```python
from build123d import *

# Parameters (mm, degrees)
SKETCH1_W            = 126
SKETCH1_H            = 76
BOSS_EXTRUDE1_DEPTH  = 13
SKETCH2_W            = 126
SKETCH2_H            = 90
BOSS_EXTRUDE2_DEPTH  = 13
FILLET1_R            = 25
SKETCH3_W            = 10
SKETCH3_H            = 25.459891015
BOSS_EXTRUDE3_DEPTH  = 10
SKETCH4_W            = 10
SKETCH4_H            = 13
CUT_EXTRUDE1_DEPTH   = 10
SKETCH8_R            = 25
BOSS_EXTRUDE4_DEPTH  = 38
SKETCH10_R           = 16
CUT_EXTRUDE3_DEPTH   = 38
BOSS_EXTRUDE8_DEPTH  = 25
SKETCH12_W           = 10
SKETCH12_H           = 10
CUT_EXTRUDE4_DEPTH   = 45
SKETCH13_R           = 8.829907476
CUT_EXTRUDE5_DEPTH   = 14
SKETCH14_R           = 7
CUT_EXTRUDE6_DEPTH   = 34
BOSS_EXTRUDE11_DEPTH = 37
CUT_EXTRUDE7_DEPTH   = 37


with BuildPart() as part:
    # Sketch1 → Boss-Extrude1 (new body)
    with BuildSketch(Plane(origin=(0, 0, 0), x_dir=(1, 0, 0), z_dir=(0, 1, 0))):
        with Locations((9.064748201, -38.597122302)):
            Rectangle(SKETCH1_W, SKETCH1_H)
    extrude(amount=BOSS_EXTRUDE1_DEPTH)

    # Sketch2 → Boss-Extrude2 (add)
    with BuildSketch(Plane(origin=(0, 0, 0.597122302), x_dir=(-1, 0, 0), z_dir=(0, 0, -1))):
        with Locations((-9.064748201, 58)):
            Rectangle(SKETCH2_W, SKETCH2_H)
    extrude(amount=-BOSS_EXTRUDE2_DEPTH)

    # Fillet1
    fillet1_edges = [part.edges().sort_by_distance(p)[0] for p in [
        (72.064748201, 103, 7.097122302),
        (-53.935251799, 103, 7.097122302),
    ]]
    fillet(fillet1_edges, radius=FILLET1_R)

    # Sketch3 → Boss-Extrude3 (add)
    with BuildSketch(Plane(origin=(0, 103, 0), x_dir=(1, 0, 0), z_dir=(0, 1, 0))):
        with Locations((9.064748201, -26.32706781)):
            Rectangle(SKETCH3_W, SKETCH3_H)
    extrude(amount=-BOSS_EXTRUDE3_DEPTH)

    # Sketch4 → Cut-Extrude1 (cut)
    with BuildSketch(Plane(origin=(0, 103, 0), x_dir=(1, 0, 0), z_dir=(0, 1, 0))):
        with Locations((9.064748201, -7.097122302)):
            Rectangle(SKETCH4_W, SKETCH4_H)
    extrude(amount=-CUT_EXTRUDE1_DEPTH, mode=Mode.SUBTRACT)

    # Sketch8 → Boss-Extrude4 (add)
    with BuildSketch(Plane.XY.offset(13.597122302)):
        with Locations((9.064748201, 45.775653821)):
            Circle(SKETCH8_R)
    extrude(amount=BOSS_EXTRUDE4_DEPTH)

    # Sketch10 → Cut-Extrude3 (cut)
    with BuildSketch(Plane.XY.offset(51.597122302)):
        with Locations((9.064748201, 45.775653821)):
            Circle(SKETCH10_R)
    extrude(amount=-CUT_EXTRUDE3_DEPTH, mode=Mode.SUBTRACT)

    # Sketch11 → Boss-Extrude8 (add)
    with BuildSketch(Plane.XY.offset(13.597122302)):
        with BuildLine():
            Line((4.064748201, 103), (-5.935251799, 103))
            Line((-5.935251799, 103), (-5.935251799, 65.775653821))
            ThreePointArc((-5.935251799, 65.775653821), (9.064748201, 70.775653821), (24.064748201, 65.775653821))
            Line((24.064748201, 65.775653821), (24.064748201, 103))
            Line((24.064748201, 103), (14.064748201, 103))
            Line((14.064748201, 103), (14.064748201, 93))
            Line((14.064748201, 93), (4.064748201, 93))
            Line((4.064748201, 93), (4.064748201, 103))
        make_face()
    extrude(amount=BOSS_EXTRUDE8_DEPTH)

    # Sketch12 → Cut-Extrude4 (cut)
    with BuildSketch(Plane.XY.offset(39.057013317)):
        with Locations((9.064748201, 98)):
            Rectangle(SKETCH12_W, SKETCH12_H)
    extrude(amount=-CUT_EXTRUDE4_DEPTH, mode=Mode.SUBTRACT)

    # Sketch13 → Cut-Extrude5 (cut)
    with BuildSketch(Plane(origin=(0, 13, 0), x_dir=(1, 0, 0), z_dir=(0, 1, 0))):
        with Locations((-34.808854568, -51.290114298)):
            Circle(SKETCH13_R)
    extrude(amount=-CUT_EXTRUDE5_DEPTH, mode=Mode.SUBTRACT)

    # Sketch14 → Cut-Extrude6 (cut)
    with BuildSketch(Plane(origin=(0, 13, 0), x_dir=(1, 0, 0), z_dir=(0, 1, 0))):
        with Locations((53.064748201, -51.597122302)):
            Circle(SKETCH14_R)
    extrude(amount=-CUT_EXTRUDE6_DEPTH, mode=Mode.SUBTRACT)

    # Sketch17 → Boss-Extrude11 (add, symmetric)
    with BuildSketch(Plane.XY.offset(51.597122302)):
        Polygon((3.660374399, 21.366787731), (13.431056495, 21.159899681), (13.431056495, 13), (3.660374399, 13), align=None)
    extrude(amount=BOSS_EXTRUDE11_DEPTH, both=True)

    # Sketch18 → Cut-Extrude7 (cut, symmetric)
    with BuildSketch(Plane(origin=(13.431056495, 0, 0), x_dir=(0, 0, -1), z_dir=(1, 0, 0))):
        Polygon((-51.597122302, 21.159899681), (-76.597122302, 13), (-88.597122302, 13), (-88.597122302, 23.683887041), align=None)
    extrude(amount=CUT_EXTRUDE7_DEPTH, both=True, mode=Mode.SUBTRACT)


solid = part.part
```
Geometry check sheet. Reference: the model listing, model coordinates, mm. A direction names the side the tool comes from. Coordinates: 2 decimals unless noted, no trailing zeros. Loops run counter-clockwise (first coordinate to the right, second up) from the corner with the lowest first, then second, coordinate; pieces in that order, holes last.
Item 1: Go/stop test with flat-tipped pins: pin 1 Ø15 at (x, y) = (20.5, 57.5) entering from +Z; pin 2 Ø3 at (x, z) = (11, 18) entering from +Y; pin 3 Ø7.5 at (y, z) = (78.5, 21) entering from -X; pin 4 Ø4 at (y, z) = (58.5, 54) entering from -X. Record where each tip stops, or that it passes through.
Item 2: Sectioned sample at A-A, the plane z = 28. Record the boundary of the cut face in (x, y), then the cut area to 3 significant figures.
Item 3: Sectioned sample at C-C, the plane z = 64. Record the boundary of the cut face in (x, y), then the cut area to 3 significant figures.
Item 4: Sectioned sample at B-B, the plane y = 54. Record the boundary of the cut face in (x, z), then the cut area to 3 significant figures.
Item 5: Release check for a two-part mould opening along Y. For faces 1 (the face through (3.66, 17, 39)), 2 (the face through (-5, 103, 15)), 3 (the face through (9, 85, 38.597)) record: released by +Y, released by -Y, zero draft, split by the parting line, or undercut.
Item 6: Thickness scan on line 1 (Y direction, x = 14.5, z = 50.5); line 2 (Y direction, x = -2.5, z = 45.5); line 3 (Z direction, x = 60, y = 66). Record the ranges inside material, lowest first.
Item 7: Sectioned sample at D-D, the plane x = -13.5. Record the boundary of the cut face in (y, z).
Item 8: Access from +Z, -Z, +X, -X, +Y, -Y to the whole of each face (thin tool, end or side, straight path). Record for faces 4 (the face through (9, 46, 13.597)), 5 (the face through (24.065, 84, 26)), 6 (the face through (9, 93, 20)).
Check result:
1. pin 1: stops at z = 51.6
1. pin 2: stops at y = 93
1. pin 3: stops at x = -5.94
1. pin 4: passes through
2. outline: (-53.94, 0) - (72.06, 0) - (72.06, 13) - (13.43, 13) - (13.43, 21.16) arc R25 ccw to (24.06, 65.78) - (24.06, 103) - (14.06, 103) - (14.06, 93) - (4.06, 93) - (4.06, 103) - (-5.94, 103) - (-5.94, 65.78) arc R25 ccw to (3.66, 21.37) - (3.66, 13) - (-53.94, 13) - close; hole circle Ø32 at (9.06, 45.78)
2. area: 3,790 mm2
3. outline: (-53.94, 0) - (72.06, 0) - (72.06, 13) - (13.43, 13) - (13.43, 17.11) - (3.66, 17.11) - (3.66, 13) - (-53.94, 13) - close
3. area: 1,680 mm2
4. outline: (-53.94, 0.6) - (72.06, 0.6) - (72.06, 13.6) - (32.67, 13.6) - (32.67, 51.6) - (22.79, 51.6) - (22.79, 13.6) - (-4.66, 13.6) - (-4.66, 51.6) - (-14.54, 51.6) - (-14.54, 13.6) - (-53.94, 13.6) - close
4. area: 2,390 mm2
5. face 1: undercut
5. face 2: released by +Y
5. face 3: zero draft
6. line 1: y = 0 to 13, 21.37 to 30.73, 60.82 to 70.18
6. line 2: y = 0 to 13, 23.61 to 34.72, 56.83 to 67.94
6. line 3: z = 0.6 to 13.6
7. outline: (0, 0.6) - (103, 0.6) - (103, 13.6) - (56.54, 13.6) - (56.54, 51.6) - (35.01, 51.6) - (35.01, 13.6) - (13, 13.6) - (13, 76.6) - (0, 76.6) - close
8. face 4: +Z
8. face 5: +Z, +X, +Y
8. face 6: +Z, -Z, +Y
